Design review of the part shown in the three views and the two pictorial views. Dimensions are in mm from the part's minimum x, y and z. A direction names the side the tool comes from. Round coordinates to 2 decimals unless told otherwise and drop trailing zeros. Order: outer loops, then holes, each group sorted by start corner. A loop starts at its lowest first (then second) coordinate and runs counter-clockwise, first axis right, second up. Notation, with made-up numbers: M -34.75,-9.5 L 11.25,-9.5 A25 cw 11.25,16.5 Z; hole C 28.25,-19.75 d7. An arc over 180 degrees is marked long. Use a Markdown table: item, result. Add a question column.
(1) Take a section at B-B (x = 6). Write out the cut boundary in (y, z), then the cut area to 3 significant figures.
(2) To check wall thickness, follow probe 1 along Z at (x, y) = (6, 13); probe 2 along Z at (x, y) = (6, 3). State the ranges of each line that lie inside material, in increasing order. Write a range as from..to.
(3) Take a section at C-C (y = 1.75). Write out the cut boundary in (x, z), then the cut area to 3 significant figures.
(4) For pin 1 (4 mm diameter, centred on x = 4.5, y = 3, fed in from -Z); pin 2 (3 mm diameter, centred on y = 8, z = 4, fed in from -X); pin 3 (5 mm diameter, centred on y = 2, z = 2, fed in from +X); pin 4 (2 mm diameter, centred on y = 8.5, z = 10.5, fed in from -X), all flat-tipped, find the tip position at first contact; note any pin that passes through.
(5) Take a section at D-D (y = 11.75). Write out the cut boundary in (x, z), then the cut area to 3 significant figures.
(6) Take a section at A-A (z = 6). Write out the cut boundary in (x, y), then the cut area to 3 significant figures.
(7) Machinability: for the marked faces 1 and 2, which of the approach directions +Z, -Z, +X, -X, +Y, -Y give a long, thin tool a straight path to every point of the face, cutting with its end or side? Answer none if there is none.
(8) The part is to be moulded in two halves that separate along Z. For the marked faces 3, 4 and 5, say which applies: released by +Z, released by -Z, zero draft, split by the parting line, or undercut.
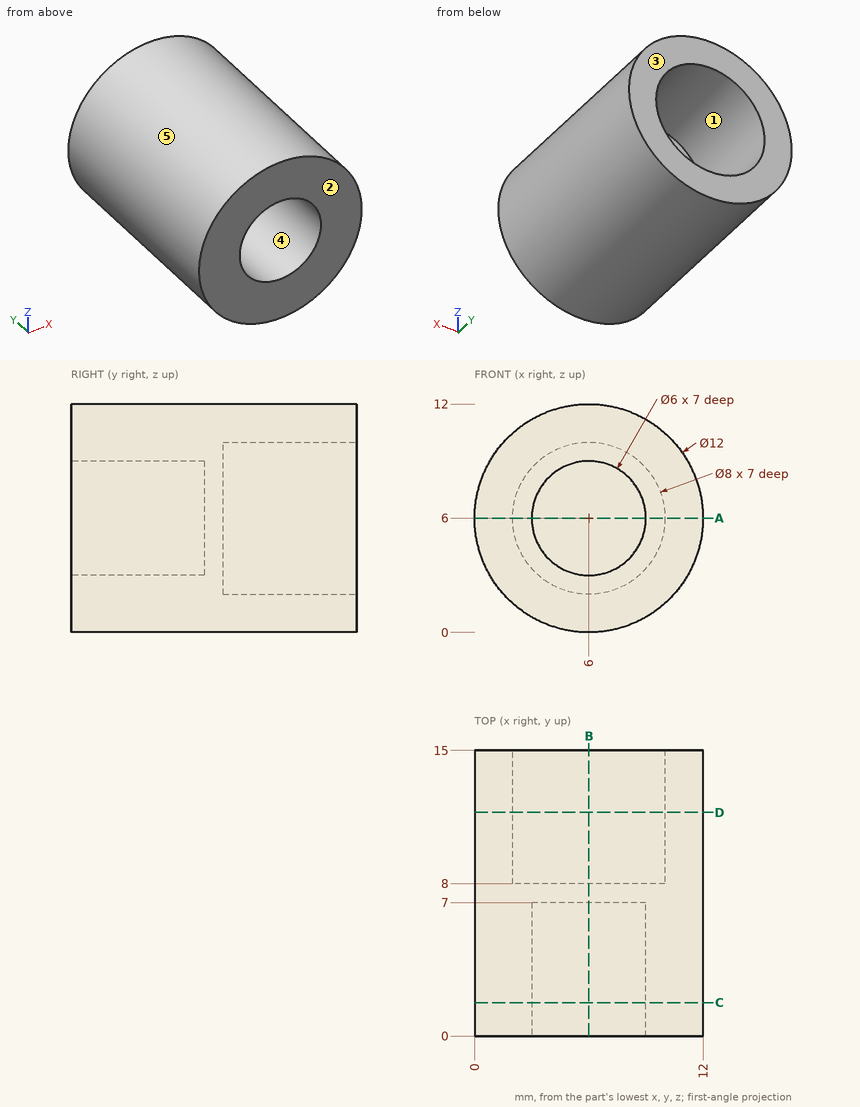
Verdict:
| question | item | result |
|---|---|---|
| 1 | outline | M 0,0 L 15,0 L 15,2 L 8,2 L 8,10 L 15,10 L 15,12 L 0,12 L 0,9 L 7,9 L 7,3 L 0,3 Z |
| 1 | area | 82.0 mm^2 |
| 2 | probe 1 | z = 0..2, 10..12 |
| 2 | probe 2 | z = 0..3, 9..12 |
| 3 | outline | C 6,6 d12; hole C 6,6 d6 |
| 3 | area | 84.8 mm^2 |
| 4 | pin 1 | stops at z = 0 |
| 4 | pin 2 | stops at x = 0.02 |
| 4 | pin 3 | stops at x = 11.81 |
| 4 | pin 4 | stops at x = 1.13 |
| 5 | outline | C 6,6 d12; hole C 6,6 d8 |
| 5 | area | 62.8 mm^2 |
| 6 | outline | M 0,0 L 3,0 L 3,7 L 9,7 L 9,0 L 12,0 L 12,15 L 10,15 L 10,8 L 2,8 L 2,15 L 0,15 Z |
| 6 | area | 82.0 mm^2 |
| 7 | face 1 | +Y |
| 7 | face 2 | +Z, -Z, +X, -X, -Y |
| 8 | face 3 | zero draft |
| 8 | face 4 | undercut |
| 8 | face 5 | split by the parting line |
